```python
from build123d import *


with BuildPart() as part:
    # Sketch1 → Revolve1 (revolve)
    with BuildSketch(Plane.XY):
        Polygon((20.574, 9.525), (20.574, 8.7376), (21.3614, 8.7376), (21.3614, 9.525), (21.6154, 9.525), (21.6154, 8.7376), (22.4028, 8.7376), (22.4028, 9.525), (22.6568, 9.525), (22.6568, 8.7376), (23.4442, 8.7376), (23.4442, 9.525), (23.6982, 9.525), (23.6982, 8.7376), (24.4856, 8.7376), (24.4856, 9.525), (24.7396, 9.525), (24.7396, 8.7376), (25.527, 8.7376), (25.527, 9.525), (25.781, 9.525), (25.781, 9.271), (26.797, 9.271), (26.797, 8.4836), (27.5844, 8.4836), (27.5844, 9.271), (27.8384, 9.271), (27.8384, 8.4836), (28.6258, 8.4836), (28.6258, 9.271), (28.8798, 9.271), (28.8798, 8.4836), (29.6672, 8.4836), (29.6672, 9.271), (29.9212, 9.271), (29.9212, 8.4836), (30.7086, 8.4836), (30.7086, 9.271), (30.9626, 9.271), (30.9626, 8.4836), (31.75, 8.4836), (31.75, 9.271), (32.004, 9.271), (32.004, 9.017), (33.02, 9.017), (33.02, 8.2296), (33.8074, 8.2296), (33.8074, 9.017), (34.0614, 9.017), (34.0614, 8.2296), (34.8488, 8.2296), (34.8488, 9.017), (35.1028, 9.017), (35.1028, 8.2296), (35.8902, 8.2296), (35.8902, 9.017), (36.1442, 9.017), (36.1442, 8.2296), (36.9316, 8.2296), (36.9316, 9.017), (37.1856, 9.017), (37.1856, 8.2296), (37.973, 8.2296), (37.973, 9.017), (38.227, 9.017), (38.227, 8.763), (39.243, 8.763), (39.243, 7.9756), (40.0304, 7.9756), (40.0304, 8.763), (40.2844, 8.763), (40.2844, 7.9756), (41.0718, 7.9756), (41.0718, 8.763), (41.3258, 8.763), (41.3258, 7.9756), (42.1132, 7.9756), (42.1132, 8.763), (42.3672, 8.763), (42.3672, 7.9756), (43.1546, 7.9756), (43.1546, 8.763), (43.4086, 8.763), (43.4086, 7.9756), (44.196, 7.9756), (44.196, 8.763), (44.45, 8.763), (44.45, 8.509), (45.466, 8.509), (45.466, 7.7216), (46.2534, 7.7216), (46.2534, 8.509), (46.5074, 8.509), (46.5074, 7.7216), (47.2948, 7.7216), (47.2948, 8.509), (47.5488, 8.509), (47.5488, 7.7216), (48.3362, 7.7216), (48.3362, 8.509), (48.5902, 8.509), (48.5902, 7.7216), (49.3776, 7.7216), (49.3776, 8.509), (49.6316, 8.509), (49.6316, 7.7216), (50.419, 7.7216), (50.419, 8.509), (50.673, 8.509), (50.673, 8.255), (51.689, 8.255), (51.689, 7.4676), (52.4764, 7.4676), (52.4764, 8.255), (52.7304, 8.255), (52.7304, 7.4676), (53.5178, 7.4676), (53.5178, 8.255), (53.7718, 8.255), (53.7718, 7.4676), (54.5592, 7.4676), (54.5592, 8.255), (54.8132, 8.255), (54.8132, 7.4676), (55.6006, 7.4676), (55.6006, 8.255), (55.8546, 8.255), (55.8546, 7.4676), (56.642, 7.4676), (56.642, 8.255), (56.896, 8.255), (56.896, 5.999988), (77.216, 5.999988), (77.216, 0), (61.976, 0), (0, 0), (0, 5.999988), (20.32, 5.999988), (20.32, 9.525), align=None)
    revolve(axis=Axis((0, 0, 0), (1, 0, 0)))


solid = part.part
```
Model file for the job. Use its own axes, mm. Coordinates: 2 decimals unless noted, no trailing zeros. Order: outer loops, then holes, each group sorted by start corner. A loop starts at its lowest first (then second) coordinate and runs counter-clockwise, first axis right, second up. Notation, with made-up numbers: (-15.75, -5) - (7.25, -5) arc R20 cw to (7.25, 15) - close; hole circle Ø3 at (17.25, -2). An arc over 180 degrees is marked (long way). Return JSON: item names as keys, results as strings. Group by question number.
1) Flat gauge pins, fed straight in: P1, Ø4, axis at x = 16.5, y = 4, coming from the +Z side; P2, Ø8, axis at x = 66.5, y = 1, coming from the -Z side; P3, Ø6, axis at x = 49, y = 5, coming from the -Z side. Where does each tip first touch, or does it go through?
2) Saw through at A-A, the plane x = 67.5. Write the cut outline in (y, z).
3) Probe line 1 (X direction, y = -6.5, z = -4); line 2 (X direction, y = -5.5, z = -4.25); line 3 (Z direction, x = 33.5, y = -3). List the from-to ranges inside material, lowest first. Write a range as from..to.
Values found:
{
 "1": {"P1": "stops at z = 5.66", "P2": "stops at z = -6", "P3": "stops at z = -8.26"},
 "2": {"outline": "circle Ø12 at (0, 0)"},
 "3": {"line 1": "x = 20.32..51.69, 52.48..52.73, 53.52..53.77, 54.56..54.81, 55.6..55.85, 56.64..56.9", "line 2": "x = 20.32..56.9", "line 3": "z = -7.66..7.66"}
}
